Geometry check sheet. Reference: drawing and pictorial views, mm from the part's lowest x, y, z. A direction names the side the tool comes from. Coordinates: 2 decimals unless noted, no trailing zeros. Write each loop counter-clockwise with the first axis right and the second up, starting at its lowest first coordinate (ties: lowest second). Pieces come first, ordered by that corner, then holes. Notation, with made-up numbers: (-29.5, 89.5) -> (27.5, 89.5) arc R23 cw to (27.5, 113.5) -> close; hole circle Ø5 at (48.5, 3.5). An arc over 180 degrees is marked (long way). Use a Markdown table: item, result.
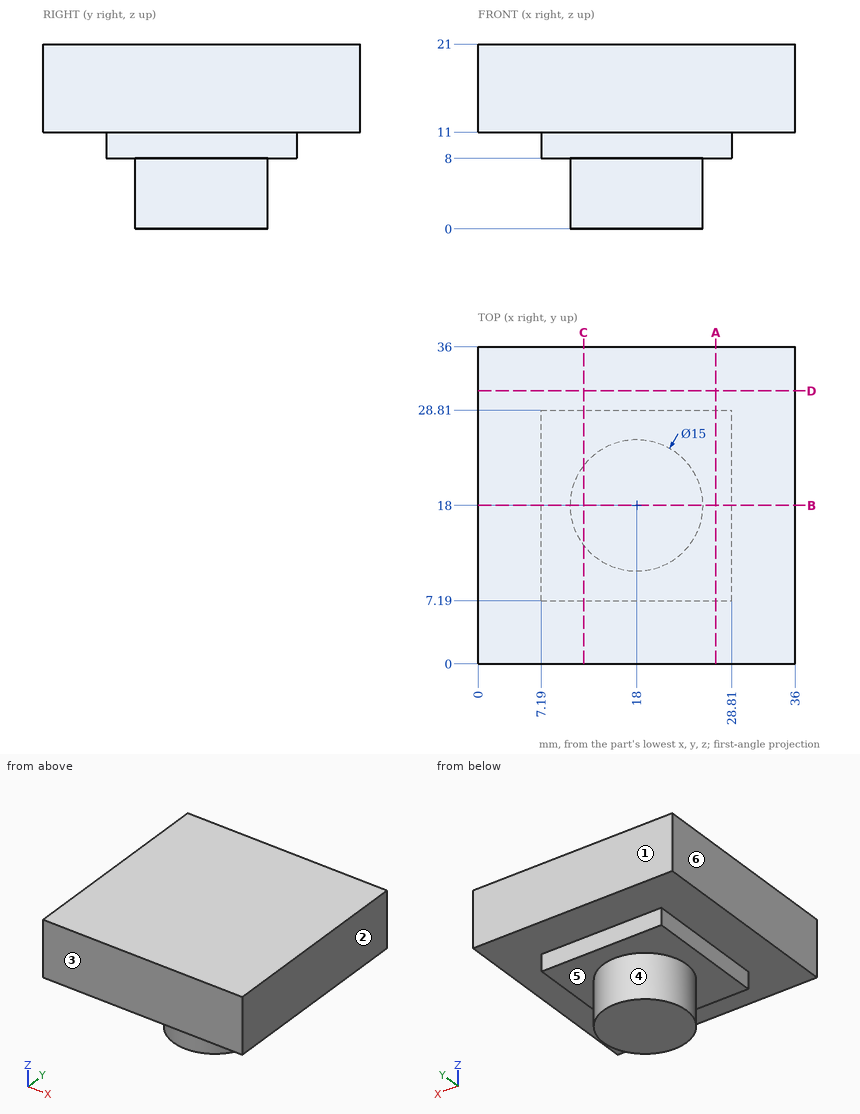
Item 1: Thickness scan on L1, parallel to Z at x = 26, y = 17.5; L2, parallel to Z at x = 11.5, y = 29.5; L3, parallel to X at y = 23, z = 7.75. Record the ranges inside material, lowest first. Write a range as [from, to].
Answer block:
| item | result |
|---|---|
| L1 | z = [8, 21] |
| L2 | z = [11, 21] |
| L3 | x = [12.41, 23.59] |
Item 2: Mould release check, pull along Y, two halves, no side actions. Record for the marked faces 1, 2, 3 and 4: +Y half, -Y half, draft (parallel to the pull), parting line (faces both ways), or undercut.
Answer block:
| item | result |
|---|---|
| face 1 | +Y half |
| face 2 | draft |
| face 3 | -Y half |
| face 4 | parting line |
Item 3: Section check D-D on y = 31. Record the boundary of the cut face in (x, z), then the cut area to 3 significant figures.
Answer block:
| item | result |
|---|---|
| outline | (0, 11) -> (36, 11) -> (36, 21) -> (0, 21) -> close |
| area | 360 mm^2 |
Item 4: Depth check by flat-ended pin: P1, Ø1, axis at y = 27, z = 9, coming from the +X side; P2, Ø1, axis at x = 13.5, z = 4.5, coming from the +Y side; P3, Ø3, axis at x = 22.5, z = 6, coming from the +Y side. Enter the tip coordinate at first touch or a pass-through.
Answer block:
| item | result |
|---|---|
| P1 | stops at x = 28.81 |
| P2 | stops at y = 24.34 |
| P3 | stops at y = 24.87 |
Item 5: Tool access check on the marked faces 5 and 6. Record the directions out of +Z, -Z, +X, -X, +Y, -Y that give a thin tool (end or side, any length) a straight path to the whole face; none if there is none.
Answer block:
| item | result |
|---|---|
| face 5 | -Z |
| face 6 | +Z, -Z, -X, +Y, -Y |
Item 6: Section check C-C on x = 12. Record the boundary of the cut face in (y, z), then the cut area to 3 significant figures.
Answer block:
| item | result |
|---|---|
| outline | (0, 11) -> (7.19, 11) -> (7.19, 8) -> (13.5, 8) -> (13.5, 0) -> (22.5, 0) -> (22.5, 8) -> (28.81, 8) -> (28.81, 11) -> (36, 11) -> (36, 21) -> (0, 21) -> close |
| area | 497 mm^2 |
Item 7: Section check B-B on y = 18. Record the boundary of the cut face in (x, z), then the cut area to 3 significant figures.
Answer block:
| item | result |
|---|---|
| outline | (0, 11) -> (7.19, 11) -> (7.19, 8) -> (10.5, 8) -> (10.5, 0) -> (25.5, 0) -> (25.5, 8) -> (28.81, 8) -> (28.81, 11) -> (36, 11) -> (36, 21) -> (0, 21) -> close |
| area | 545 mm^2 |
Item 8: Section check A-A on x = 27. Record the boundary of the cut face in (y, z).
Answer block:
| item | result |
|---|---|
| outline | (0, 11) -> (7.19, 11) -> (7.19, 8) -> (28.81, 8) -> (28.81, 11) -> (36, 11) -> (36, 21) -> (0, 21) -> close |
